The listing builds one solid part. Answer for the finished solid, in the listing's coordinates (mm). Face numbers are marked on the shaded views. A direction names the side the tool comes from. Give positions to 0.01 mm unless a question says otherwise; leave off trailing zeros. Loops run counter-clockwise (first coordinate to the right, second up) from the corner with the lowest first, then second, coordinate; pieces in that order, holes last.
Item 1: Section C-C, the plane z = 1 is taken. Give the vertices of the cut face in (x, y), and give its area (3 significant figures).
Item 2: Section D-D, the plane x = -8.5 is taken. Give the vertices of the cut face in (y, z), and give its area (3 significant figures).
Item 3: A tool of negligible diameter and unlimited length cuts with its end or side. For the marked faces 1, 2 and 3, from which of +Z, -Z, +X, -X, +Y, -Y can it reach the whole face along a straight path? Write none if from no direction.
Item 4: Consider line 1 along Y through (x, z) = (-15.5, 1); line 2 along X through (y, z) = (9, 3.75); line 3 along Z through (x, y) = (1, 11.75). Determine where each line is inside the solid, lowest interval first.
Item 5: Each of these flat-tipped pins is pushed along its axis until it touches: pin 1 Ø0.5 at (x, z) = (-19.5, 4) entering from -Y; pin 2 Ø1.8 at (x, z) = (2, 2.5) entering from -Y; pin 3 Ø0.7 at (x, y) = (-12, 18.5) entering from +Z. Where does it stop, or does it pass through?
Item 6: Section B-B, the plane y = 18.5 is taken. Give the vertices of the cut face in (x, z) (3 decimals).
Item 7: Section A-A, the plane x = -19.5 is taken. Give the vertices of the cut face in (y, z) (3 decimals).
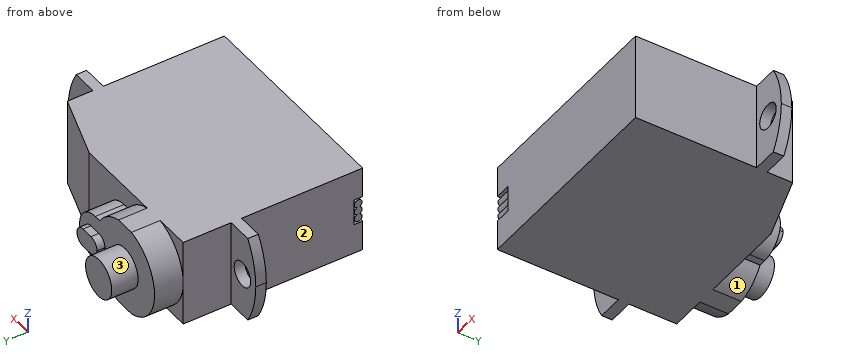
from build123d import *

# Parameters (mm, degrees)
SKETCH1_W           = 20.25
SKETCH1_H           = 8.45
BOSS_EXTRUDE1_DEPTH = 12.7
SKETCH2_W           = 8.45
SKETCH2_H           = 1.016
BOSS_EXTRUDE2_DEPTH = 3.61
CUT_EXTRUDE1_REACH  = 27.353
SKETCH3_R           = 1.205
SKETCH4_W           = 20.25
SKETCH4_H           = 8.45
BOSS_EXTRUDE3_DEPTH = 4.6228
CHAMFER1_SIZE       = 2.159
CHAMFER1_SIZE2      = 6.477
SKETCH5_R           = 1.9177
BOSS_EXTRUDE4_DEPTH = 5.3086
SKETCH6_R           = 1.9177
BOSS_EXTRUDE5_DEPTH = 2.7686
BOSS_EXTRUDE6_DEPTH = 0.762
SKETCH8_W           = 2.54
SKETCH8_H           = 0.8636
CUT_EXTRUDE2_DEPTH  = 1.6002
SKETCH9_R           = 0.381
BOSS_EXTRUDE9_DEPTH = 1.6002


with BuildPart() as part:
    # Sketch1 → Boss-Extrude1 (new body)
    with BuildSketch(Plane(origin=(0, 0, 0), x_dir=(1, 0, 0), z_dir=(0, 1, 0))):
        with Locations((-10.125, -4.225)):
            Rectangle(SKETCH1_W, SKETCH1_H)
    extrude(amount=BOSS_EXTRUDE1_DEPTH)

    # Sketch2 → Boss-Extrude2 (add)
    with BuildSketch(Plane(origin=(0, 0, 0), x_dir=(0, 0, -1), z_dir=(1, 0, 0))):
        with Locations((-4.225, 12.192)):
            Rectangle(SKETCH2_W, SKETCH2_H)
    boss_extrude2 = extrude(amount=BOSS_EXTRUDE2_DEPTH)

    # Sketch3 → Cut-Extrude1 (cut, up to next)
    with BuildSketch(Plane(origin=(0, 12.7, 0), x_dir=(1, 0, 0), z_dir=(0, 1, 0)), mode=Mode.PRIVATE) as cut_extrude1_sk1:
        with BuildLine():
            ThreePointArc((3.61, -4.225), (3.312097542, -6.417003935), (2.44, -8.45))
            Line((2.44, -8.45), (3.61, -8.45))
            Line((3.61, -8.45), (3.61, -4.225))
        make_face()
    cut_extrude1_tool1 = extrude(cut_extrude1_sk1.sketch, amount=-CUT_EXTRUDE1_REACH, mode=Mode.PRIVATE) & part.part
    # Sketch3 → Cut-Extrude1 (cut, up to next)
    with BuildSketch(Plane(origin=(0, 12.7, 0), x_dir=(1, 0, 0), z_dir=(0, 1, 0)), mode=Mode.PRIVATE) as cut_extrude1_sk2:
        with BuildLine():
            ThreePointArc((2.44, 0), (3.312097542, -2.032996065), (3.61, -4.225))
            Line((3.61, -4.225), (3.61, 0))
            Line((3.61, 0), (2.44, 0))
        make_face()
    cut_extrude1_tool2 = extrude(cut_extrude1_sk2.sketch, amount=-CUT_EXTRUDE1_REACH, mode=Mode.PRIVATE) & part.part
    # Sketch3 → Cut-Extrude1 (cut, up to next)
    with BuildSketch(Plane(origin=(0, 12.7, 0), x_dir=(1, 0, 0), z_dir=(0, 1, 0)), mode=Mode.PRIVATE) as cut_extrude1_sk3:
        with Locations(Location((1.655, -4.225, 0), (0, 0, 270))):
            Circle(SKETCH3_R)
    cut_extrude1_tool3 = extrude(cut_extrude1_sk3.sketch, amount=-CUT_EXTRUDE1_REACH, mode=Mode.PRIVATE) & part.part
    cut_extrude1_1 = cut_extrude1_tool1.solids().sort_by_distance((3.263745, 12.7, 7.409386))[0]
    add(cut_extrude1_1, mode=Mode.SUBTRACT)
    cut_extrude1_2 = cut_extrude1_tool2.solids().sort_by_distance((3.263745, 12.7, 1.040614))[0]
    add(cut_extrude1_2, mode=Mode.SUBTRACT)
    cut_extrude1_3 = cut_extrude1_tool3.solids().sort_by_distance((1.655, 12.7, 4.225))[0]
    add(cut_extrude1_3, mode=Mode.SUBTRACT)
    cut_extrude1 = cut_extrude1_1 + cut_extrude1_2 + cut_extrude1_3  # Cut-Extrude1 as one shape, for the pattern or mirror that repeats it

    # Mirror1: Boss-Extrude2, Cut-Extrude1 across plane
    add(boss_extrude2.mirror(Plane(origin=(-10.125, 0, 0), x_dir=(0, 0, 1), z_dir=(1, 0, 0))))
    add(cut_extrude1.mirror(Plane(origin=(-10.125, 0, 0), x_dir=(0, 0, 1), z_dir=(1, 0, 0))), mode=Mode.SUBTRACT)

    # Sketch4 → Boss-Extrude3 (add)
    with BuildSketch(Plane(origin=(0, 12.7, 0), x_dir=(1, 0, 0), z_dir=(0, 1, 0))):
        with Locations((-10.125, -4.225)):
            Rectangle(SKETCH4_W, SKETCH4_H)
    extrude(amount=BOSS_EXTRUDE3_DEPTH)

    # Chamfer1
    chamfer1_edges = [part.edges().sort_by_distance(p)[0] for p in [
        (0, 17.3228, 4.225),
    ]]
    chamfer1_side = [part.faces().sort_by_distance(p)[0] for p in [
        (0, 15.0114, 4.225),
    ]]
    chamfer(chamfer1_edges, length=CHAMFER1_SIZE, length2=CHAMFER1_SIZE2, reference=chamfer1_side[0])

    # Sketch5 → Boss-Extrude4 (add)
    with BuildSketch(Plane(origin=(0, 17.3228, 0), x_dir=(1, 0, 0), z_dir=(0, 1, 0))):
        with Locations(Location((-15.9193, -4.225, 0), (0, 0, 90))):
            Circle(SKETCH5_R)
    extrude(amount=BOSS_EXTRUDE4_DEPTH)

    # Sketch6 → Boss-Extrude5 (add)
    # profile 1 of 2: a face of its own
    with BuildSketch(Plane(origin=(0, 17.3228, 0), x_dir=(1, 0, 0), z_dir=(0, 1, 0))):
        with BuildLine():
            Line((-11.5759, -1.9263), (-12.249021972, -1.9263))
            ThreePointArc((-12.249021972, -1.9263), (-11.5886, -4.225), (-12.249021972, -6.5237))
            Line((-12.249021972, -6.5237), (-11.5759, -6.5237))
            ThreePointArc((-11.5759, -6.5237), (-9.2772, -4.225), (-11.5759, -1.9263))
        make_face()
    # profile 2 of 2: a face of its own
    with BuildSketch(Plane(origin=(0, 17.3228, 0), x_dir=(1, 0, 0), z_dir=(0, 1, 0))):
        with BuildLine():
            Line((-14.968333392, 0), (-16.870266608, 0))
            ThreePointArc((-16.870266608, 0), (-20.25, -4.225), (-16.870266608, -8.45))
            Line((-16.870266608, -8.45), (-14.968333392, -8.45))
            ThreePointArc((-14.968333392, -8.45), (-13.415975527, -7.758883002), (-12.249021972, -6.5237))
            ThreePointArc((-12.249021972, -6.5237), (-11.5886, -4.225), (-12.249021972, -1.9263))
            ThreePointArc((-12.249021972, -1.9263), (-13.415975527, -0.691116998), (-14.968333392, 0))
        make_face()
        with Locations(Location((-15.9193, -4.225, 0), (0, 0, 270))):
            Circle(SKETCH6_R, mode=Mode.SUBTRACT)
    extrude(amount=BOSS_EXTRUDE5_DEPTH)

    # Sketch7 → Boss-Extrude6 (add)
    with BuildSketch(Plane(origin=(0, 20.0914, 0), x_dir=(1, 0, 0), z_dir=(0, 1, 0))):
        with BuildLine():
            Line((-10.0392, -4.225), (-12.9856, -4.225))
            ThreePointArc((-12.9856, -4.225), (-12.724790977, -4.854648681), (-12.095142296, -5.115457704))
            Line((-12.095142296, -5.115457704), (-10.929657704, -5.115457704))
            ThreePointArc((-10.929657704, -5.115457704), (-10.300009023, -4.854648681), (-10.0392, -4.225))
        make_face()
        with BuildLine():
            ThreePointArc((-12.095142296, -3.334542296), (-12.724790977, -3.595351319), (-12.9856, -4.225))
            Line((-12.9856, -4.225), (-10.0392, -4.225))
            ThreePointArc((-10.0392, -4.225), (-10.300009023, -3.595351319), (-10.929657704, -3.334542296))
            Line((-10.929657704, -3.334542296), (-12.095142296, -3.334542296))
        make_face()
    extrude(amount=BOSS_EXTRUDE6_DEPTH)

    # Sketch8 → Cut-Extrude2 (cut)
    with BuildSketch(Plane.ZY.offset(20.25)):
        with Locations((4.225, 0.4318)):
            Rectangle(SKETCH8_W, SKETCH8_H)
    extrude(amount=-CUT_EXTRUDE2_DEPTH, mode=Mode.SUBTRACT)

    # Sketch9 → Boss-Extrude9 (add)
    with BuildSketch(Plane.ZY.offset(18.6498)):
        with Locations((4.961591366, 0.4318)):
            Circle(SKETCH9_R)
        with Locations((4.225, 0.435366491)):
            Circle(SKETCH9_R)
        with Locations((3.488408634, 0.4318)):
            Circle(SKETCH9_R)
    extrude(amount=BOSS_EXTRUDE9_DEPTH)


solid = part.part
Worked answers:
1. outline: (-23.2, 11.68) - (-20.25, 11.68) - (-20.25, 0) - (0, 0) - (0, 11.68) - (2.95, 11.68) - (2.95, 12.7) - (0, 12.7) - (0, 15.16) - (-6.48, 17.32) - (-13.03, 17.32) - (-13.03, 20.09) - (-18.81, 20.09) - (-18.81, 17.32) - (-20.25, 17.32) - (-20.25, 12.7) - (-23.2, 12.7) - close
1. area: 366 mm2
2. outline: (0, 0) - (17.32, 0) - (17.32, 8.45) - (0, 8.45) - close
2. area: 146 mm2
3. face 1: -Z, +X, +Y
3. face 2: +Z, -Z, -X, -Y
3. face 3: +Y
4. line 1: y = 0 to 20.09
4. line 2: x = -20.25 to 0
4. line 3: z = 0 to 3.21, 5.24 to 8.45
5. pin 1: stops at y = 0.05
5. pin 2: stops at y = 11.68
5. pin 3: stops at z = 6.68
6. outline: (-16.87, 0) - (-14.968, 0) arc R4.331 ccw to (-12.249, 1.926) - (-11.576, 1.926) arc R2.299 ccw to (-11.576, 6.524) - (-12.249, 6.524) arc R4.331 ccw to (-14.968, 8.45) - (-16.87, 8.45) arc R4.331 ccw to start
7. outline: (0, 0) - (17.323, 0) - (17.323, 1.789) - (20.091, 1.789) - (20.091, 6.661) - (17.323, 6.661) - (17.323, 8.45) - (0, 8.45) - (0, 5.495) - (0.864, 5.495) - (0.864, 2.955) - (0, 2.955) - close; (0.336, 3.857) arc R0.381 ccw (long way) to (0.531, 3.856) arc R0.381 ccw to (0.531, 4.594) arc R0.381 ccw (long way) to (0.336, 4.593) arc R0.381 ccw to start
